The listing builds one solid part. Answer for the finished solid, in the listing's coordinates (mm). Coordinates: 2 decimals unless noted, no trailing zeros. Write each loop counter-clockwise with the first axis right and the second up, starting at its lowest first coordinate (ties: lowest second). Pieces come first, ordered by that corner, then holes. Notation, with made-up numbers: M 47,45.25 L 70,45.25 A27 ccw 70,81.25 Z; hole C 76.25,-5 d8. An arc over 180 degrees is marked long. Answer as CSV lines item,"result".
```python
from build123d import *

# Parameters (mm, degrees)
SKETCH1_W            = 375
SKETCH1_H            = 200
SKETCH1_R            = 20
BASE_FLANGE1_DEPTH   = 1.5875
M5_CLEARANCE_HOLE1_D = 5.8
MIRROR2_COPY_1_D     = 5.8
FILLET1_R            = 2
FILLET2_R            = 2
FILLET3_R            = 2
FILLET4_R            = 2
SKETCH9_W            = 103
SKETCH9_H            = 20.5
CUT_EXTRUDE1_DEPTH   = 10
FILLET5_R            = 2
FILLET6_R            = 2
SKETCH10_R           = 20
BOSS_EXTRUDE1_DEPTH  = 1.5875
SKETCH11_R           = 36
CUT_EXTRUDE2_DEPTH   = 10


# Sheet-metal steps are written as plain solids
with BuildPart() as part:
    # Sketch1 → Base-Flange1 (new body)
    with BuildSketch(Plane(origin=(0, 0, 0), x_dir=(0, 0, -1), z_dir=(1, 0, 0))):
        Rectangle(SKETCH1_W, SKETCH1_H)
        Circle(SKETCH1_R, mode=Mode.SUBTRACT)
    extrude(amount=-BASE_FLANGE1_DEPTH)

    # M5 Clearance Hole1 (through all)
    with Locations(Plane.ZY.offset(1.5875)):
        with Locations((177.5, 90)):
            m5_clearance_hole1 = Hole(M5_CLEARANCE_HOLE1_D / 2)

    # Mirror1: M5 Clearance Hole1 across plane
    add(m5_clearance_hole1.mirror(Plane.XY), mode=Mode.SUBTRACT)

    # Mirror2: M5 Clearance Hole1 across plane
    add(m5_clearance_hole1.mirror(Plane.ZX), mode=Mode.SUBTRACT)

    # Mirror2 copy 1 (through all)
    with Locations(Plane(origin=(-1.5875, 0, 0), x_dir=(0, 0, -1), z_dir=(-1, 0, 0))):
        with Locations((177.5, 90)):
            Hole(MIRROR2_COPY_1_D / 2)

    # Fillet1
    fillet1_edges = [part.edges().sort_by_distance(p)[0] for p in [
        (-0.79375, -100, -187.5),
    ]]
    fillet(fillet1_edges, radius=FILLET1_R)

    # Fillet2
    fillet2_edges = [part.edges().sort_by_distance(p)[0] for p in [
        (-0.79375, 100, -187.5),
    ]]
    fillet(fillet2_edges, radius=FILLET2_R)

    # Fillet3
    fillet3_edges = [part.edges().sort_by_distance(p)[0] for p in [
        (-0.79375, 100, 187.5),
    ]]
    fillet(fillet3_edges, radius=FILLET3_R)

    # Fillet4
    fillet4_edges = [part.edges().sort_by_distance(p)[0] for p in [
        (-0.79375, -100, 187.5),
    ]]
    fillet(fillet4_edges, radius=FILLET4_R)

    # Sketch9 → Cut-Extrude1 (cut)
    with BuildSketch(Plane(origin=(0, 0, 0), x_dir=(0, 0, -1), z_dir=(1, 0, 0))):
        with Locations((0, -89.75)):
            Rectangle(SKETCH9_W, SKETCH9_H)
    extrude(amount=-CUT_EXTRUDE1_DEPTH, mode=Mode.SUBTRACT)

    # Fillet5
    fillet5_edges = [part.edges().sort_by_distance(p)[0] for p in [
        (-0.79375, -100, -51.5),
    ]]
    fillet(fillet5_edges, radius=FILLET5_R)

    # Fillet6
    fillet6_edges = [part.edges().sort_by_distance(p)[0] for p in [
        (-0.79375, -100, 51.5),
    ]]
    fillet(fillet6_edges, radius=FILLET6_R)

    # Sketch10 → Boss-Extrude1 (add)
    with BuildSketch(Plane(origin=(0, 0, 0), x_dir=(0, 0, -1), z_dir=(1, 0, 0))):
        Circle(SKETCH10_R)
    extrude(amount=-BOSS_EXTRUDE1_DEPTH)

    # Sketch11 → Cut-Extrude2 (cut)
    with BuildSketch(Plane(origin=(0, 0, 0), x_dir=(0, 0, -1), z_dir=(1, 0, 0))):
        with Locations((0, -5.28)):
            Circle(SKETCH11_R)
    extrude(amount=-CUT_EXTRUDE2_DEPTH, mode=Mode.SUBTRACT)


solid = part.part
```
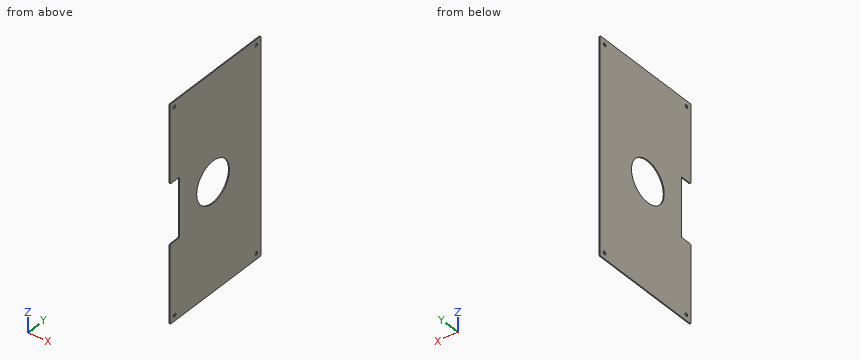
Q1. Flat-ended cylindrical pins translate along their axes: pin 1 Ø3.5 at (y, z) = (90, 177.5) entering from -X; pin 2 Ø9.5 at (y, z) = (-90, 177.5) entering from -X. Find the tip coordinate at first contact, or state that the pin passes through.
Output:
pin 1,"through"
pin 2,"x = -1.59"
Q2. Straight lines are drawn through the part: line 1 (Y direction, x = -0.6, z = 177.5); line 2 (Y direction, x = -0.45, z = 0); line 3 (Z direction, x = -0.25, y = -38.5). For each, find the intervals that lie inside material, in ascending order.
Output:
line 1,"-100 to -92.9, -87.1 to 87.1, 92.9 to 100"
line 2,"-79.5 to -41.28, 30.72 to 100"
line 3,"-187.5 to -13.87, 13.87 to 187.5"
Q3. Find section A-A (z = 0). Give the vertices of the cut face in (x, y), and give its area (3 significant figures).
Output:
outline,"M -1.59,-79.5 L 0,-79.5 L 0,-41.28 L -1.59,-41.28 Z; M -1.59,30.72 L 0,30.72 L 0,100 L -1.59,100 Z"
area,"171 mm2"
Q4. Find section B-B (x = -1). Give the vertices of the cut face in (y, z).
Output:
outline,"M -100,-185.5 A2 ccw -98,-187.5 L 98,-187.5 A2 ccw 100,-185.5 L 100,185.5 A2 ccw 98,187.5 L -98,187.5 A2 ccw -100,185.5 L -100,53.5 A2 ccw -98,51.5 L -79.5,51.5 L -79.5,-51.5 L -98,-51.5 A2 ccw -100,-53.5 Z; hole C -90,-177.5 d5.8; hole C -90,177.5 d5.8; hole C -5.28,0 d72; hole C 90,-177.5 d5.8; hole C 90,177.5 d5.8"
